Here's the drawing with two shaded views (mm, measured from the low corner). I have some questions. A direction names the side the tool comes from. Coordinates: 2 decimals unless noted, no trailing zeros. Order: outer loops, then holes, each group sorted by start corner. A loop starts at its lowest first (then second) coordinate and runs counter-clockwise, first axis right, second up. Notation, with made-up numbers: (-8, 40) - (7, 40) arc R27 ccw to (7, 65) - close; hole circle Ø3 at (22.5, -33.5). An arc over 180 degrees is marked (long way). Answer as a JSON object with one key per item and string values. Group by question number.
(1) Will these pins go through, and if not, where does the flat tip stop? P1, Ø16, axis at x = 8, z = 24.5, coming from the -Y side; P2, Ø5, axis at x = 20.5, z = 13.5, coming from the -Y side; P3, Ø10, axis at x = 4.5, z = 14, coming from the +Y side; P4, Ø8, axis at x = 5, y = 35, coming from the -Z side.
(2) Imagine slicing it at C-C, the plane y = 62.3. Write out the boundary of the cut face in (x, z).
(3) Imagine slicing it at D-D, the plane z = 20. Write out the boundary of the cut face in (x, y), and give its area (3 significant figures).
(4) Which directions (+Z, -Z, +X, -X, +Y, -Y) give clear straight access to the entire face, cutting with the end or side of a thin tool? Please do the marked faces 1, 2 and 3.
(5) Imagine slicing it at B-B, the plane y = 21.15. Write out the boundary of the cut face in (x, z), and give its area (3 significant figures).
(6) We'd pull the mould along Y, two halves only. Please class the marked faces 4, 5 and 6: pulls with the +Y half, pulls with the -Y half, needs draft (parallel to the pull), parting line crosses it, or undercut.
(7) Please list where these lines run through material, in increasing order: probe 1 along Z at (x, y) = (22.5, 45.95); probe 2 along Y at (x, z) = (7.5, 2.1); probe 3 along X at (y, z) = (21, 1).
(8) Imagine slicing it at A-A, the plane x = 22.5. Write out the boundary of the cut face in (y, z), and give its area (4 significant figures).
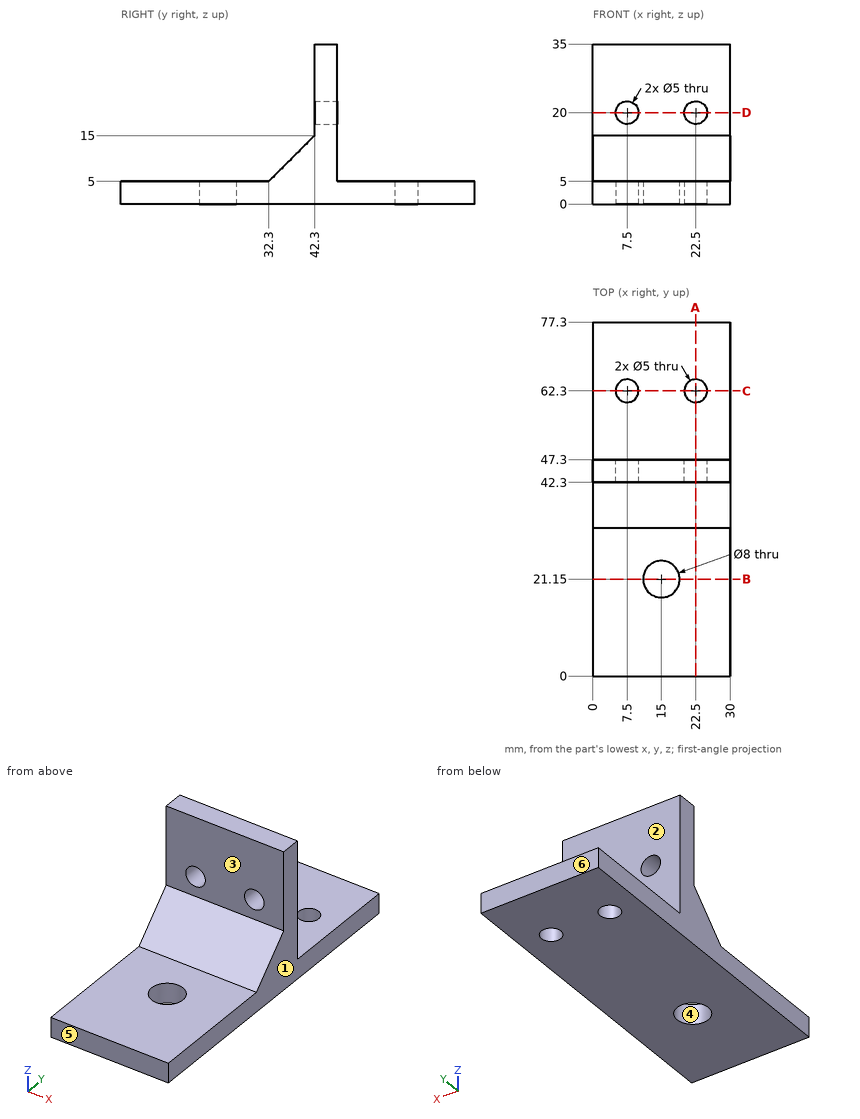
Result set:
{
 "1": {"P1": "stops at y = 42.3", "P2": "stops at y = 38.3", "P3": "stops at y = 47.3", "P4": "stops at z = 0"},
 "2": {"outline": "(0, 0) - (5, 0) - (5, 5) - (0, 5) - close; (10, 0) - (20, 0) - (20, 5) - (10, 5) - close; (25, 0) - (30, 0) - (30, 5) - (25, 5) - close"},
 "3": {"outline": "(0, 42.3) - (5, 42.3) - (5, 47.3) - (0, 47.3) - close; (10, 42.3) - (20, 42.3) - (20, 47.3) - (10, 47.3) - close; (25, 42.3) - (30, 42.3) - (30, 47.3) - (25, 47.3) - close", "area": "100 mm^2"},
 "4": {"face 1": "+Z, -Z, +X, +Y, -Y", "face 2": "+Z, +X, -X, +Y", "face 3": "+Z, +X, -X, -Y"},
 "5": {"outline": "(0, 0) - (11, 0) - (11, 5) - (0, 5) - close; (19, 0) - (30, 0) - (30, 5) - (19, 5) - close", "area": "110 mm^2"},
 "6": {"face 4": "undercut", "face 5": "pulls with the -Y half", "face 6": "pulls with the +Y half"},
 "7": {"probe 1": "z = 0 to 17.5, 22.5 to 35", "probe 2": "y = 0 to 59.8, 64.8 to 77.3", "probe 3": "x = 0 to 11, 19 to 30"},
 "8": {"outline": "(0, 0) - (59.8, 0) - (59.8, 5) - (47.3, 5) - (47.3, 17.5) - (42.3, 17.5) - (42.3, 15) - (32.3, 5) - (0, 5) - close; (42.3, 22.5) - (47.3, 22.5) - (47.3, 35) - (42.3, 35) - close; (64.8, 0) - (77.3, 0) - (77.3, 5) - (64.8, 5) - close", "area": "536.5 mm^2"}
}
